from build123d import *

# Parameters (mm, degrees)
F1_DEPTH = 25.4


with BuildPart() as f1:
    # F0 (on Front) → F1 (new body)
    with BuildSketch(Plane.XZ):
        with BuildLine():
            ThreePointArc((-25.270923, 80.211686), (-16.685877, 69.118101), (-6.356709, 78.609094))
            ThreePointArc((-6.356709, 78.609094), (-6.370167, 79.115242), (-6.410502, 79.61996))
            ThreePointArc((-6.410502, 79.61996), (-15.583019, 88.129409), (-25.270923, 80.211686))
        make_face()
        with BuildLine():
            ThreePointArc((-6.410502, 79.61996), (-6.370167, 79.115242), (-6.356709, 78.609094))
            ThreePointArc((-6.356709, 78.609094), (-16.685877, 69.118101), (-25.270923, 80.211686))
            Line((-25.270923, 80.211686), (-32.456549, 43.534504))
            ThreePointArc((-32.456549, 43.534504), (-16.797117, 56.357165), (-1.268692, 43.376162))
            Line((-1.268692, 43.376162), (-6.410502, 79.61996))
        make_face()
        with BuildLine():
            Line((-1.07973, 42.044204), (-1.268692, 43.376162))
            ThreePointArc((-1.268692, 43.376162), (-16.797117, 56.357165), (-32.456549, 43.534504))
            Line((-32.456549, 43.534504), (-32.456549, 37.430235))
            ThreePointArc((-32.456549, 37.430235), (-16.444514, 24.613281), (-1.155568, 38.284701))
            ThreePointArc((-1.155568, 38.284701), (-1.040974, 39.380881), (-1.002714, 40.482369))
            ThreePointArc((-1.002714, 40.482369), (-1.02198, 41.264236), (-1.07973, 42.044204))
        make_face()
        with BuildLine():
            ThreePointArc((-1.07973, 42.044204), (-1.160095, 42.712186), (-1.268692, 43.376162))
            Line((-1.268692, 43.376162), (-1.07973, 42.044204))
        make_face()
        with BuildLine():
            Line((-32.456549, 37.430235), (-32.456549, 43.534504))
            ThreePointArc((-32.456549, 43.534504), (-32.752714, 40.482369), (-32.456549, 37.430235))
        make_face()
        with BuildLine():
            ThreePointArc((-1.155568, 38.284701), (-16.444514, 24.613281), (-32.456549, 37.430235))
            Line((-32.456549, 37.430235), (-25.390898, -24.178508))
            ThreePointArc((-25.390898, -24.178508), (-22.914287, -16.16678), (-15.338004, -12.572156))
            ThreePointArc((-15.338004, -12.572156), (-14.236036, -12.598485), (-13.14301, -12.741041))
            Line((-13.14301, -12.741041), (-4.059813, -13.439911))
            Line((-4.059813, -13.439911), (-1.155568, 38.284701))
        make_face()
        with BuildLine():
            ThreePointArc((-15.338004, -12.572156), (-22.914287, -16.16678), (-25.390898, -24.178508))
            ThreePointArc((-25.390898, -24.178508), (-21.951109, -30.7895), (-14.976151, -33.413874))
            Line((-14.976151, -33.413874), (-14.393512, -33.394246))
            ThreePointArc((-14.393512, -33.394246), (-7.441734, -30.130543), (-4.612501, -22.990906))
            ThreePointArc((-4.612501, -22.990906), (-7.024118, -16.323273), (-13.14301, -12.741041))
            Line((-13.14301, -12.741041), (-15.338004, -12.572156))
        make_face()
        with BuildLine():
            Line((30.023281, -16.062297), (-4.059813, -13.439911))
            Line((-4.059813, -13.439911), (-13.14301, -12.741041))
            ThreePointArc((-13.14301, -12.741041), (-7.024118, -16.323273), (-4.612501, -22.990906))
            ThreePointArc((-4.612501, -22.990906), (-7.441734, -30.130543), (-14.393512, -33.394246))
            Line((-14.393512, -33.394246), (29.681615, -31.909406))
            ThreePointArc((29.681615, -31.909406), (21.478706, -23.805312), (30.023281, -16.062297))
        make_face()
        with BuildLine():
            Line((-14.393512, -33.394246), (-14.976151, -33.413874))
            ThreePointArc((-14.976151, -33.413874), (-14.684694, -33.408134), (-14.393512, -33.394246))
        make_face()
        with BuildLine():
            ThreePointArc((37.351861, -23.976406), (35.238329, -18.583327), (30.023281, -16.062297))
            ThreePointArc((30.023281, -16.062297), (21.478706, -23.805312), (29.681615, -31.909406))
            ThreePointArc((29.681615, -31.909406), (35.120728, -29.493769), (37.351861, -23.976406))
        make_face()
    extrude(amount=F1_DEPTH)


solid = f1.part
Check sheet for the modelled part. Datum: model origin and axes. Units: mm. A direction names the side the tool comes from. Round coordinates to 2 decimals unless told otherwise and drop trailing zeros. Loops run counter-clockwise (first coordinate to the right, second up) from the corner with the lowest first, then second, coordinate; pieces in that order, holes last. Notation, with made-up numbers: M 75,-4 L 111,-4 A5 ccw 111,1 Z; hole C 48,-18 d6. An arc over 180 degrees is marked long. One line per item, written item: value.
(1) Sectioned sample at C-C, the plane x = 7. Record the cut outline in (y, z).
Computed values:
outline: M -25.4,-32.67 L 0,-32.67 L 0,-14.29 L -25.4,-14.29 Z
(2) Thickness scan on line 1 (X direction, y = -19, z = 3.5); line 2 (Z direction, x = 2, y = -6.5); line 3 (Z direction, x = -0.5, y = -21). Record the ranges inside material, lowest first.
Computed values:
line 1: x = -28.57 to -3.11
line 2: z = -32.84 to -13.91
line 3: z = -32.93 to -13.71
(3) Sectioned sample at B-B, the plane z = 47. Record the cut outline in (x, y).
Computed values:
outline: M -31.78,-25.4 L -1.78,-25.4 L -1.78,0 L -31.78,0 Z
(4) Depth check by flat-ended pin: pin 1 Ø12 at (y, z) = (-7.5, 69) entering from +X; pin 2 Ø5 at (y, z) = (-5.5, 29.5) entering from -X; pin 3 Ø8 at (x, y) = (-9.5, -11) entering from +Z. Enter the tip coordinate at first touch or a pass-through.
Computed values:
pin 1: stops at x = -4.05
pin 2: stops at x = -31.83
pin 3: stops at z = 87.83
(5) Access from +Z, -Z, +X, -X, +Y, -Y to the whole of each face (thin tool, end or side, straight path). Record for faces 1 (the face through (-1.04, -12.52, 39.37)), 2 (the face through (-14, 0, 15)).
Computed values:
face 1: +X, +Y, -Y
face 2: +Z, -Z, +X, -X, +Y
